Check sheet for the modelled part. Datum: model origin and axes. Units: mm. Face numbers are marked on the shaded views. A direction names the side the tool comes from. Give positions to 0.01 mm unless a question says otherwise; leave off trailing zeros. Loops run counter-clockwise (first coordinate to the right, second up) from the corner with the lowest first, then second, coordinate; pieces in that order, holes last. Notation, with made-up numbers: (61, 16) -> (80, 16) arc R8 cw to (80, 26) -> close; hole circle Ø8 at (53.25, 63). An arc over 180 degrees is marked (long way). Write each question's results on one line, items separated by ' | '. Start each with the question number.
1. Tool access check on the marked faces 1 and 2. Record the directions out of +Z, -Z, +X, -X, +Y, -Y that give a thin tool (end or side, any length) a straight path to the whole face; none if there is none.
2. Cross-section at A-A on x = 42.5. Record the boundary of the cut face in (y, z), and give its area (3 significant figures).
3. Material ranges on L1, parallel to Y at x = 50.25, z = -8; L2, parallel to X at y = -8, z = -7.25; L3, parallel to Z at x = 49.75, y = 29, recorded low to high. Write a range as from..to.
4. Cross-section at D-D on z = -10. Record the boundary of the cut face in (x, y), and give its area (3 significant figures).
5. Cross-section at B-B on z = -17.5. Record the boundary of the cut face in (x, y).
6. Cross-section at C-C on x = 48.5. Record the boundary of the cut face in (y, z), and give its area (3 significant figures).
7. Gauge pin test, flat ends, axial feed: pin 1 Ø10 at (x, z) = (50.5, -1.5) entering from -Y; pin 2 Ø3 at (x, z) = (50.5, -19) entering from +Y; pin 3 Ø5 at (x, y) = (44.5, 40) entering from +Z. Record the tip position at first contact, or that the pin passes through.
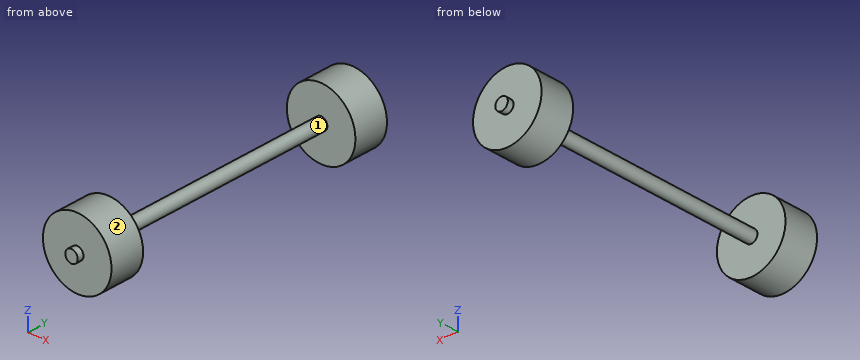
from build123d import *

# Parameters (mm, degrees)
CYLINDER002001001002_R             = 11
CYLINDER002001001002_DEPTH         = 11
CYLINDER002001001002_ROLL_ANGLE    = 90
CYLINDER002001001002001_R          = 11
CYLINDER002001001002001_DEPTH      = 11
CYLINDER002001001002001_ROLL_ANGLE = 90
CYLINDER002001002001_R             = 2
CYLINDER002001002001_DEPTH         = 100
CYLINDER002001002001_ROLL_ANGLE    = -90


with BuildPart() as wheel006:
    # Cylinder002001001002 → Cylinder002001001002 (new body)
    with BuildSketch(Plane.XY):
        Circle(CYLINDER002001001002_R)
    extrude(amount=CYLINDER002001001002_DEPTH)


with BuildPart() as wheel006_1:
    # Cylinder002001001002 roll: moved
    add(wheel006.part.rotate(Axis((0, 0, 0), (1, 0, 0)), CYLINDER002001001002_ROLL_ANGLE))


with BuildPart() as wheel006_2:
    # Cylinder002001001002 placement: moved
    add(wheel006_1.part.moved(Location((20, 78, 14))))


with BuildPart() as wheel007:
    # Cylinder002001001002001 → Cylinder002001001002001 (new body)
    with BuildSketch(Plane.XY):
        Circle(CYLINDER002001001002001_R)
    extrude(amount=CYLINDER002001001002001_DEPTH)


with BuildPart() as wheel007_1:
    # Cylinder002001001002001 roll: moved
    add(wheel007.part.rotate(Axis((0, 0, 0), (1, 0, 0)), CYLINDER002001001002001_ROLL_ANGLE))


with BuildPart() as wheel007_2:
    # Cylinder002001001002001 placement: moved
    add(wheel007_1.part.moved(Location((20, -7, 14))))


with BuildPart() as obj1:
    # Cylinder002001002001 → Cylinder002001002001 (new body)
    with BuildSketch(Plane.XY):
        Circle(CYLINDER002001002001_R)
    extrude(amount=CYLINDER002001002001_DEPTH)


with BuildPart() as obj1_1:
    # Cylinder002001002001 roll: moved
    add(obj1.part.rotate(Axis((0, 0, 0), (1, 0, 0)), CYLINDER002001002001_ROLL_ANGLE))


with BuildPart() as obj1_2:
    # Cylinder002001002001 placement: moved
    add(obj1_1.part.moved(Location((20, -20, 14))))

    # Fusion002001002002002: union Wheel006, Wheel007
    add(wheel006_2.part)
    add(wheel007_2.part)


with BuildPart() as obj1_3:
    # Fusion002001002002002 placement: moved
    add(obj1_2.part.moved(Location((28.5, 0, -24))))


solid = obj1_3.part
Geometry says:
1) face 1: none | face 2: +Y, -Y
2) outline: (-18, -19.22) -> (-7, -19.22) -> (-7, -0.78) -> (-18, -0.78) -> close; (67, -19.22) -> (78, -19.22) -> (78, -0.78) -> (67, -0.78) -> close | area: 406 mm^2
3) L1: -18..-7, 67..78 | L2: 37.85..59.15 | L3: -11.56..-8.44
4) outline: (37.5, -18) -> (46.5, -18) -> (46.5, -20) -> (50.5, -20) -> (50.5, -18) -> (59.5, -18) -> (59.5, -7) -> (50.5, -7) -> (50.5, 67) -> (59.5, 67) -> (59.5, 78) -> (50.5, 78) -> (50.5, 80) -> (46.5, 80) -> (46.5, 78) -> (37.5, 78) -> (37.5, 67) -> (46.5, 67) -> (46.5, -7) -> (37.5, -7) -> close | area: 796 mm^2
5) outline: (40.45, -18) -> (56.55, -18) -> (56.55, -7) -> (40.45, -7) -> close; (40.45, 67) -> (56.55, 67) -> (56.55, 78) -> (40.45, 78) -> close
6) outline: (-20, -12) -> (-18, -12) -> (-18, -21) -> (-7, -21) -> (-7, -12) -> (67, -12) -> (67, -21) -> (78, -21) -> (78, -12) -> (80, -12) -> (80, -8) -> (78, -8) -> (78, 1) -> (67, 1) -> (67, -8) -> (-7, -8) -> (-7, 1) -> (-18, 1) -> (-18, -8) -> (-20, -8) -> close | area: 796 mm^2
7) pin 1: y = -18 | pin 2: y = 78 | pin 3: z = -8.68
